from build123d import *

# Parameters (mm, degrees)
F1_DEPTH = 165.1
F2_R     = 4.064
F3_DEPTH = 43.18


with BuildPart() as f1:
    # F0 (on Front) → F1 (new body)
    with BuildSketch(Plane.XZ):
        Polygon((0, 38.1), (0, 0), (38.1, 0), (38.1, 19.05), (19.05, 19.05), (19.05, 38.1), align=None)
    extrude(amount=F1_DEPTH)

    # F2 (on face) → F3 (join)
    with BuildSketch(Plane.XY.offset(19.05)):
        with Locations((28.575, -25.4)):
            Circle(F2_R)
        with Locations((28.575, -139.7)):
            Circle(F2_R)
    extrude(amount=F3_DEPTH)


solid = f1.part
Can you work these out from the model? Positions are in its coordinate system, mm. A direction names the side the tool comes from. Give positions to 0.01 mm unless a question says otherwise; leave off trailing zeros. Order: outer loops, then holes, each group sorted by start corner. A loop starts at its lowest first (then second) coordinate and runs counter-clockwise, first axis right, second up. Notation, with made-up numbers: M -12,77 L 32,77 A4 cw 32,82 Z; hole C 64,-4.75 d6. An arc over 180 degrees is marked long. Use one line per item in the form item = value.
Item 1: Thinking about a two-plate mould opening in Y: for faces 6 (the cylindrical face through (30.45, -143.305, 40.338)), 7 (the flat face through (15, -165.1, 15)), 8 (the flat face through (29, -25, 62.23)), which applies, pulls with the +Y half, pulls with the -Y half, needs draft (parallel to the pull), parting line crosses it, or undercut?
Values follow:
face_6 = undercut
face_7 = pulls with the -Y half
face_8 = needs draft
Item 2: For faces 1 (the flat face through (19.05, -81, 28)), 2 (the flat face through (10, -81, 38.1)), 3 (the flat face through (15, 0, 15)), 4 (the cylindrical face through (32.329, -26.957, 40.338)), 5 (the flat face through (38.1, -81, 9)), which set-ups out of +Z, -Z, +X, -X, +Y, -Y let a thin tool reach every point of the face, with its end or its side?
Values follow:
face_1 = +Z, +Y, -Y
face_2 = +Z, -X, +Y, -Y
face_3 = +Z, -Z, +X, -X, +Y
face_4 = +Z
face_5 = +Z, -Z, +X, +Y, -Y
Item 3: If we section it at A-A, the plane y = -139.7: Write out the boundary of the cut face in (x, z).
Values follow:
outline = M 0,0 L 38.1,0 L 38.1,19.05 L 32.64,19.05 L 32.64,62.23 L 24.51,62.23 L 24.51,19.05 L 19.05,19.05 L 19.05,38.1 L 0,38.1 Z
Item 4: Will these pins go through, and if not, where does the flat tip stop? pin 1 Ø1 at (y, z) = (-22, 48.5) entering from +X; pin 2 Ø9.5 at (y, z) = (-119, 27.5) entering from +X; pin 3 Ø10 at (y, z) = (-26, 48) entering from +X.
Values follow:
pin_1 = 31.42
pin_2 = 19.05
pin_3 = 32.64
Item 5: If we section it at B-B, the plane z = 52: Write out the boundary of the cut face in (x, y) (3 decimals).
Values follow:
outline = C 28.575,-139.7 d8.128; C 28.575,-25.4 d8.128
Item 6: If we section it at D-D, the plane y = -84: Write out the boundary of the cut face in (x, z).
Values follow:
outline = M 0,0 L 38.1,0 L 38.1,19.05 L 19.05,19.05 L 19.05,38.1 L 0,38.1 Z
Item 7: If we section it at C-C, the plane x = 22: Write out the boundary of the cut face in (y, z).
Values follow:
outline = M -165.1,0 L 0,0 L 0,19.05 L -165.1,19.05 Z
Item 8: If I drill on line 1 along X through (y, z) = (-25.5, 31.5); line 2 along Z through (x, y) = (17, -59); line 3 along Z through (x, y) = (27, -67), over which ranges is the centre line in solid material (lowest first)? Write a range as [from, to].
Values follow:
line_1 = [0, 19.05], [24.51, 32.64]
line_2 = [0, 38.1]
line_3 = [0, 19.05]
